```python
from build123d import *

# Parameters (mm, degrees)
EXTRUDE_THIN1_DEPTH = 1365.25
FILLET1_R           = 1.27


with BuildPart() as part:
    # Sketch1 → Extrude-Thin1 (new body)
    with BuildSketch(Plane.XY):
        with BuildLine():
            Line((0, 0), (-31.75, 0))
            Line((-31.75, 0), (-31.75, 53.975))
            Line((-31.75, 53.975), (-36.5125, 53.975))
            Line((-36.5125, 53.975), (-36.5125, 57.15))
            ThreePointArc((-36.5125, 57.15), (-41.002628061, 59.009871939), (-42.8625, 63.5))
            Line((-42.8625, 63.5), (-44.45, 63.5))
            Line((-44.45, 63.5), (-44.45, 92.075))
            Line((-44.45, 92.075), (-31.75, 92.075))
            Line((-31.75, 92.075), (-31.75, 136.525))
            Line((-31.75, 136.525), (0, 136.525))
            Line((0, 136.525), (0, 135.255))
            Line((0, 135.255), (-30.48, 135.255))
            Line((-30.48, 135.255), (-30.48, 90.805))
            Line((-30.48, 90.805), (-43.18, 90.805))
            Line((-43.18, 90.805), (-43.18, 64.77))
            Line((-43.18, 64.77), (-41.43118885, 64.77))
            ThreePointArc((-41.43118885, 64.77), (-40.104602448, 59.907897552), (-35.2425, 58.58131115))
            Line((-35.2425, 58.58131115), (-35.2425, 55.245))
            Line((-35.2425, 55.245), (-30.48, 55.245))
            Line((-30.48, 55.245), (-30.48, 1.27))
            Line((-30.48, 1.27), (0, 1.27))
            Line((0, 1.27), (0, 0))
        make_face()
    extrude(amount=-EXTRUDE_THIN1_DEPTH)

    # Fillet1
    fillet1_edges = [part.edges().sort_by_distance(p)[0] for p in [
        (-30.48, 90.805, -682.625),
        (-41.43118885, 64.77, -682.625),
        (-35.2425, 58.58131115, -682.625),
        (-30.48, 55.245, -682.625),
        (-31.75, 0, -682.625),
        (-36.5125, 53.975, -682.625),
        (-44.45, 63.5, -682.625),
        (-44.45, 92.075, -682.625),
        (-31.75, 136.525, -682.625),
    ]]
    fillet(fillet1_edges, radius=FILLET1_R)


solid = part.part
```
For this review, take the finished solid that the model builds, in its own axes (mm). A direction names the side the tool comes from. Coordinates: 2 decimals unless noted, no trailing zeros. Write each loop counter-clockwise with the first axis right and the second up, starting at its lowest first coordinate (ties: lowest second). Pieces come first, ordered by that corner, then holes.
(1) The part is to be moulded in two halves that separate along Y. For faces 1 (the face through (-15, 1.27, -673)), 2 (the face through (-31.75, 113, -673)), 3 (the face through (-43.18, 78, -673)), 4 (the face through (-15, 136.525, -673)), say which applies: +Y half, -Y half, draft (parallel to the pull), parting line (faces both ways), or undercut.
(2) For pin 1 Ø1.5 at (y, z) = (18.5, -964) entering from -X; pin 2 Ø3 at (x, z) = (-33.5, -905.5) entering from +Y (3 decimals); pin 3 Ø12.5 at (x, z) = (-40, -806.5) entering from -Y (3 decimals), all flat-tipped, find the tip position at first contact; note any pin that passes through.
(3) Add section C-C on y = 79. Give the boundary of the cut face in (x, z), then the cut area to 3 significant figures.
(4) Add section A-A on x = -23.5. Give the boundary of the cut face in (y, z) (3 decimals).
(5) Wall thickness on probe 1 along Y at (x, z) = (-6.5, -1087) (3 decimals); probe 2 along Y at (x, z) = (-34, -463.5) (3 decimals); probe 3 along X at (y, z) = (78, -974): over which ranges is each line inside the solid? List them lowest first.
(6) Tool access review of faces 5 (the face through (-31.75, 27, -673)), 6 (the face through (-44.45, 78, -673)), 7 (the face through (-15, 135.255, -673)): name each direction out of +Z, -Z, +X, -X, +Y, -Y from which nothing blocks a thin tool from reaching the whole face with its end or side.
Answer sheet:
1. face 1: undercut
1. face 2: draft
1. face 3: undercut
1. face 4: +Y half
2. pin 1: stops at x = -31.75
2. pin 2: stops at y = 92.075
2. pin 3: stops at y = 53.975
3. outline: (-44.45, -1365.25) - (-43.18, -1365.25) - (-43.18, 0) - (-44.45, 0) - close
3. area: 1,730 mm2
4. outline: (0, -1365.25) - (1.27, -1365.25) - (1.27, 0) - (0, 0) - close; (135.255, -1365.25) - (136.525, -1365.25) - (136.525, 0) - (135.255, 0) - close
5. probe 1: y = 0 to 1.27, 135.255 to 136.525
5. probe 2: y = 53.975 to 55.245, 90.805 to 92.075
5. probe 3: x = -44.45 to -43.18
6. face 5: +Z, -Z, -X, -Y
6. face 6: +Z, -Z, -X, +Y, -Y
6. face 7: +Z, -Z, +X
